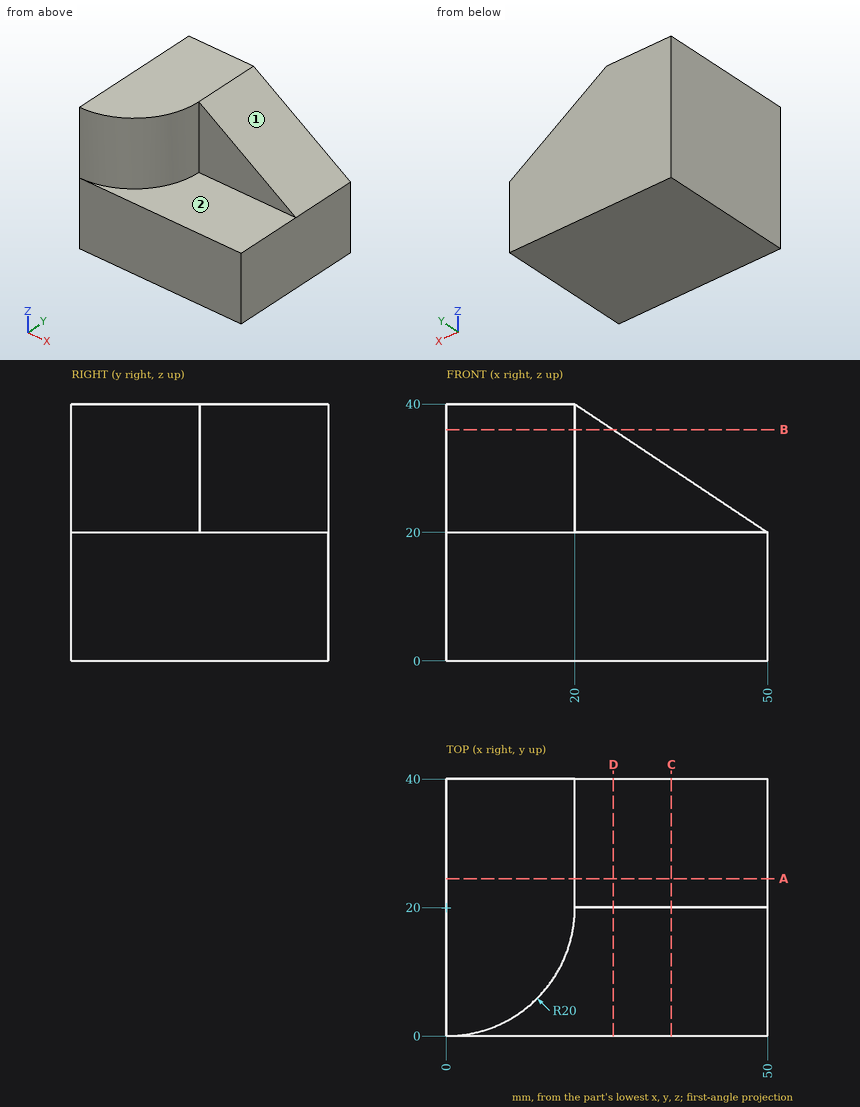
Job drawing, mm, ordinate dimensions from the low corner. One solid piece. A direction names the side the tool comes from. Round coordinates to 2 decimals unless told otherwise and drop trailing zeros. Write each loop counter-clockwise with the first axis right and the second up, starting at its lowest first coordinate (ties: lowest second). Pieces come first, ordered by that corner, then holes. Notation, with made-up numbers: (12.5, 9) -> (47.5, 9) arc R17 cw to (47.5, 42) -> close; hole circle Ø1 at (16.5, 4). An arc over 180 degrees is marked (long way). Answer as a JSON object with one key per item and string values.
(1) Probe probe 1 along Y at (x, z) = (43, 22); probe 2 along Z at (x, y) = (39, 11); probe 3 along X at (y, z) = (11.5, 31.5). List the from-to ranges inside material, lowest first. Write a range as [from, to].
Reported:
{"probe 1": "y = [20, 40]", "probe 2": "z = [0, 20]", "probe 3": "x = [0, 18.1]"}
(2) Pin check, flat tips, straight feed: P1, Ø1.5, axis at x = 44.5, y = 8, coming from the +Z side; P2, Ø2, axis at y = 6.5, z = 23, coming from the +X side; P3, Ø6, axis at x = 34, z = 33, coming from the -Y side. Stop position of each tip, or through.
Reported:
{"P1": "stops at z = 20", "P2": "stops at x = 15.61", "P3": "stops at y = 20"}
(3) Band-saw the part on A-A, the plane y = 24.5. List the corners of the cut face in (x, z), then the cut area to 3 significant figures.
Reported:
{"outline": "(0, 0) -> (50, 0) -> (50, 20) -> (20, 40) -> (0, 40) -> close", "area": "1,700 mm^2"}
(4) Which spindle directions (+Z, -Z, +X, -X, +Y, -Y) get a long thin tool onto all of the face, cutting with end or side? Do the marked faces 1 and 2. Say none if no direction does.
Reported:
{"face 1": "+Z, +X, +Y, -Y", "face 2": "+Z, +X, -Y"}
(5) Band-saw the part on D-D, the plane x = 26. List the corners of the cut face in (y, z), then the cut area to 3 significant figures.
Reported:
{"outline": "(0, 0) -> (40, 0) -> (40, 36) -> (20, 36) -> (20, 20) -> (0, 20) -> close", "area": "1,120 mm^2"}
(6) Band-saw the part on C-C, the plane x = 35. List the corners of the cut face in (y, z), then the cut area to 3 significant figures.
Reported:
{"outline": "(0, 0) -> (40, 0) -> (40, 30) -> (20, 30) -> (20, 20) -> (0, 20) -> close", "area": "1,000 mm^2"}
(7) Band-saw the part on B-B, the plane z = 36. List the corners of the cut face in (x, y).
Reported:
{"outline": "(0, 0) arc R20 ccw to (20, 20) -> (26, 20) -> (26, 40) -> (0, 40) -> close"}
